For this review, use the dimensioned drawing (mm, ordinates from the lowest corner) and the shaded views. Round coordinates to 2 decimals unless told otherwise and drop trailing zeros. Write each loop counter-clockwise with the first axis right and the second up, starting at its lowest first coordinate (ties: lowest second). Pieces come first, ordered by that corner, then holes. Notation, with made-up numbers: (41, 48.25) - (75, 48.25) arc R31 cw to (75, 81.25) - close; hole circle Ø9 at (36, -26.5). An arc over 180 degrees is marked (long way). Write each question's results on one line, items separated by ' | '.
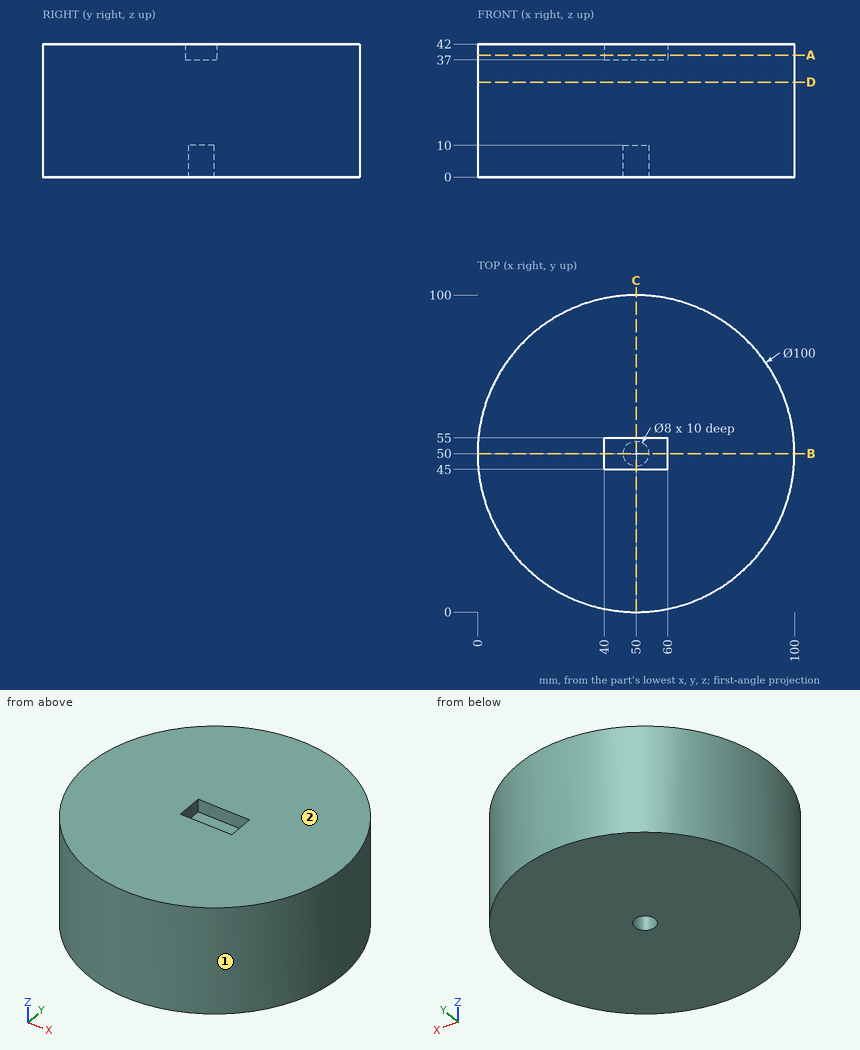
Q1. We need section D-D (z = 30). State the section outline as (x, y) points.
Evaluation:
outline: circle Ø100 at (50, 50)
Q2. For probe 1 along Y at (x, z) = (50, 7); probe 2 along Y at (x, z) = (28.5, 30); probe 3 along X at (y, z) = (35, 27), list the stretches that pass through material, from the lowest coordinate up.
Evaluation:
probe 1: y = 0 to 46, 54 to 100 | probe 2: y = 4.86 to 95.14 | probe 3: x = 2.3 to 97.7
Q3. Insertion check: P1, Ø3, axis at x = 51, y = 51, coming from the +Z side; P2, Ø10.5, axis at x = 50, y = 50, coming from the +Z side; P3, Ø1.5, axis at x = 49.5, z = 39, coming from the +Y side; P4, Ø2, axis at y = 16.5, z = 4, coming from the -X side. Each pin has a flat end and moves straight along its axis. Give the tip position at first contact, or say it passes through.
Evaluation:
P1: stops at z = 37 | P2: stops at z = 42 | P3: stops at y = 100 | P4: stops at x = 12
Q4. We need section B-B (y = 50). State the section outline as (x, z) points.
Evaluation:
outline: (0, 0) - (46, 0) - (46, 10) - (54, 10) - (54, 0) - (100, 0) - (100, 42) - (60, 42) - (60, 37) - (40, 37) - (40, 42) - (0, 42) - close
Q5. The part is to be moulded in two halves that separate along X. For the marked faces 1 and 2, say which applies: released by +X, released by -X, zero draft, split by the parting line, or undercut.
Evaluation:
face 1: split by the parting line | face 2: zero draft
Q6. We need section C-C (x = 50). State the section outline as (y, z) points, plus the area to 3 significant figures.
Evaluation:
outline: (0, 0) - (46, 0) - (46, 10) - (54, 10) - (54, 0) - (100, 0) - (100, 42) - (55, 42) - (55, 37) - (45, 37) - (45, 42) - (0, 42) - close | area: 4,070 mm^2
Q7. We need section A-A (z = 38.5). State the section outline as (x, y) points.
Evaluation:
outline: circle Ø100 at (50, 50); hole (40, 45) - (60, 45) - (60, 55) - (40, 55) - close
